```python
from build123d import *

# Parameters (mm, degrees)
F0_W     = 25
F0_H     = 25
F1_DEPTH = 17
F3_DEPTH = 16
F4_R     = 3.5
F5_DEPTH = 4


with BuildPart() as f1:
    # F0 (on Top) → F1 (new body)
    with BuildSketch(Plane.XY):
        Rectangle(F0_W, F0_H)
    extrude(amount=F1_DEPTH)

    # F2 (on face) → F3 (cut)
    with BuildSketch(Plane.XY.offset(17)):
        Polygon((-12.5, -12.5), (0, -12.5), (12.5, -12.5), (12.5, 8.5), (-12.5, 8.5), align=None)
    extrude(amount=-F3_DEPTH, mode=Mode.SUBTRACT)

    # F4 (on face) → F5 (cut, through all)
    with BuildSketch(Plane(origin=(0, 12.5, 0), x_dir=(-1, 0, 0), z_dir=(0, 1, 0))):
        with Locations((0, 9)):
            Circle(F4_R)
    extrude(amount=-F5_DEPTH, mode=Mode.SUBTRACT)


solid = f1.part
```
Here's how the part is built. I have some questions about the finished solid (model axes, mm). A direction names the side the tool comes from. Give positions to 0.01 mm unless a question says otherwise; leave off trailing zeros. Loops run counter-clockwise (first coordinate to the right, second up) from the corner with the lowest first, then second, coordinate; pieces in that order, holes last. Notation, with made-up numbers: M -38,73 L -25,73 A13 ccw -25,81 Z; hole C 69.5,42 d8. An arc over 180 degrees is marked long. Return JSON: item names as keys, results as strings.
Item 1: Please list where these lines run through material, in increasing order: line 1 (Z direction, x = 0, y = 9.6); line 2 (Y direction, x = -4.5, z = 10.5); line 3 (Z direction, x = 3, y = 2.25).
A:
{"line 1": "z = 0 to 5.5, 12.5 to 17", "line 2": "y = 8.5 to 12.5", "line 3": "z = 0 to 1"}
Item 2: Imagine slicing it at A-A on x = 0. List the corners of the cut face in (y, z) for me, then the cut area to 3 significant figures.
A:
{"outline": "M -12.5,0 L 12.5,0 L 12.5,5.5 L 8.5,5.5 L 8.5,1 L -12.5,1 Z; M 8.5,12.5 L 12.5,12.5 L 12.5,17 L 8.5,17 Z", "area": "61.0 mm^2"}
Item 3: Imagine slicing it at C-C on y = 9.25. List the corners of the cut face in (x, z) for me, then the cut area to 3 significant figures.
A:
{"outline": "M -12.5,0 L 12.5,0 L 12.5,17 L -12.5,17 Z; hole C 0,9 d7", "area": "387 mm^2"}
Item 4: Thinking about a two-plate mould opening in X: for faces 3 (the cylindrical face through (0.759, 10.528, 5.583)), 4 (the flat face through (-12.5, 9, 6)), 5 (the flat face through (-3, 12.5, 6)), which applies, released by +X, released by -X, zero draft, split by the parting line, or undercut?
A:
{"face 3": "undercut", "face 4": "released by -X", "face 5": "zero draft"}
Item 5: Imagine slicing it at D-D on x = -9.5. List the corners of the cut face in (y, z) for me, then the cut area to 3 significant figures.
A:
{"outline": "M -12.5,0 L 12.5,0 L 12.5,17 L 8.5,17 L 8.5,1 L -12.5,1 Z", "area": "89.0 mm^2"}
Item 6: Imagine slicing it at B-B on z = 9. List the corners of the cut face in (x, y) for me, then the cut area to 3 significant figures.
A:
{"outline": "M -12.5,8.5 L -3.5,8.5 L -3.5,12.5 L -12.5,12.5 Z; M 3.5,8.5 L 12.5,8.5 L 12.5,12.5 L 3.5,12.5 Z", "area": "72.0 mm^2"}
Item 7: I'm going to push flat-ended pins straight in: pin 1 Ø1.5 at (x, z) = (-5, 10) entering from -Y; pin 2 Ø10 at (x, z) = (-1, 7) entering from +Y; pin 3 Ø10.5 at (x, y) = (-5, -6) entering from +Z. Where does each tip first touch, or does it pass through?
A:
{"pin 1": "stops at y = 8.5", "pin 2": "stops at y = 12.5", "pin 3": "stops at z = 1"}
Item 8: On a 3-axis mill with a long thin cutter (end or side, diameter ignored), from which of +Z, -Z, +X, -X, +Y, -Y can I reach the whole of each face in a straight line? I mean faces 1 (the flat face through (12.5, 9, 6)), 2 (the flat face through (0, 8.5, 13)). Say none if no direction works.
A:
{"face 1": "+Z, -Z, +X, +Y, -Y", "face 2": "+Z, +X, -X, -Y"}
